Geometry check sheet. Reference: drawing and pictorial views, mm from the part's lowest x, y, z. A direction names the side the tool comes from. Round coordinates to 2 decimals unless told otherwise and drop trailing zeros. Loops run counter-clockwise (first coordinate to the right, second up) from the corner with the lowest first, then second, coordinate; pieces in that order, holes last. Notation, with made-up numbers: M 11,52.25 L 45,52.25 A24 ccw 45,78.25 Z; hole C -25.75,1.25 d7. An arc over 180 degrees is marked long. One line per question, with ' | ' between items. Start each with the question number.
(1) Section check A-A (z = 45). Record the boundary of the cut face in (x, y).
(2) Thickness scan on probe 1 along Y at (x, z) = (88, 51); probe 2 along X at (y, z) = (33, 61.5); probe 3 along Z at (x, y) = (54, 34.5). Record the ranges inside material, lowest first. Write a range as [from, to].
(3) Section check B-B (y = 38.1). Record the boundary of the cut face in (x, z) (1 decimal).
(4) Section check C-C (x = 23.5). Record the boundary of the cut face in (y, z).
(5) Section check D-D (y = 69.5). Record the boundary of the cut face in (x, z).
(6) Tool access check on the marked faces 4 and 5. Record the directions out of +Z, -Z, +X, -X, +Y, -Y that give a thin tool (end or side, any length) a straight path to the whole face; none if there is none.
(7) Draft check along X on the marked faces 1, 2 and 3. Enter one of: +X half, -X half, draft (parallel to the pull), parting line (faces both ways), or undercut.
(8) Go/stop test with a flat-tipped pin: P1, Ø2.5, axis at y = 13.64, z = 9.47, coming from the -X side. Record where the tip stops, or that it passes through.
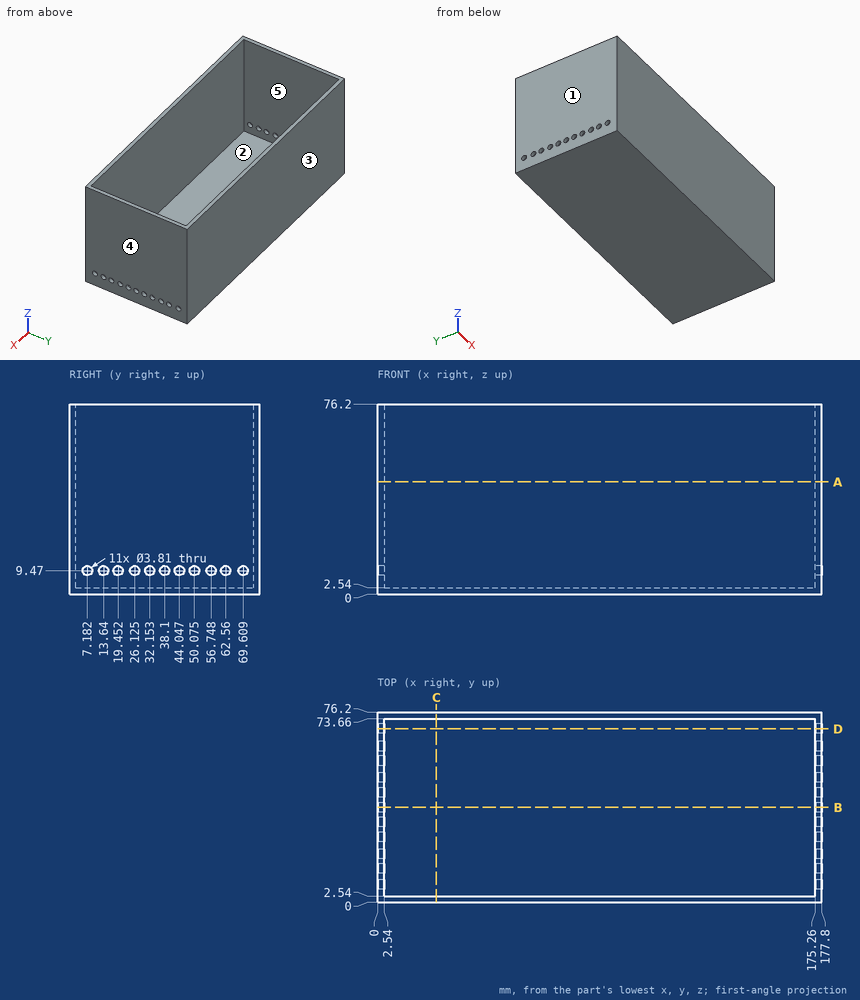
The answers:
1) outline: M 0,0 L 177.8,0 L 177.8,76.2 L 0,76.2 Z; hole M 2.54,2.54 L 175.26,2.54 L 175.26,73.66 L 2.54,73.66 Z
2) probe 1: [0, 2.54], [73.66, 76.2] | probe 2: [0, 2.54], [175.26, 177.8] | probe 3: [0, 2.54]
3) outline: M 0,0 L 177.8,0 L 177.8,7.6 L 175.3,7.6 L 175.3,2.5 L 2.5,2.5 L 2.5,7.6 L 0,7.6 Z; M 0,11.4 L 2.5,11.4 L 2.5,76.2 L 0,76.2 Z; M 175.3,11.4 L 177.8,11.4 L 177.8,76.2 L 175.3,76.2 Z
4) outline: M 0,0 L 76.2,0 L 76.2,76.2 L 73.66,76.2 L 73.66,2.54 L 2.54,2.54 L 2.54,76.2 L 0,76.2 Z
5) outline: M 0,0 L 177.8,0 L 177.8,7.57 L 175.26,7.57 L 175.26,2.54 L 2.54,2.54 L 2.54,7.57 L 0,7.57 Z; M 0,11.37 L 2.54,11.37 L 2.54,76.2 L 0,76.2 Z; M 175.26,11.37 L 177.8,11.37 L 177.8,76.2 L 175.26,76.2 Z
6) face 4: +Z, -Z, +X, +Y, -Y | face 5: +Z
7) face 1: -X half | face 2: undercut | face 3: draft
8) P1: through
